Can you work these out from the model? Positions are in its coordinate system, mm. A direction names the side the tool comes from. Round coordinates to 2 decimals unless told otherwise and drop trailing zeros. Write item = value, one per line. Start each with the question number.
1) For faces 1 (the face through (247.476, 9.578, 6.084)), 2 (the face through (77.476, 9.578, 6.084)), which set-ups out of +Z, -Z, +X, -X, +Y, -Y let a thin tool reach every point of the face, with its end or its side?
2) If I drill on line 1 (Y direction, x = 140, z = 6), over which ranges is the centre line in solid material (lowest first)?
3) Thinking about a two-plate mould opening in Z: for faces 3 (the face through (222.558, 9.672, 6.084)), 4 (the face through (123, 5, 12)), which applies, +Z half, -Z half, draft (parallel to the pull), parting line (faces both ways), or undercut?
4) I'm going to push flat-ended pins straight in: pin 1 (0.8 mm diameter, centred on x = 240, z = 3.5, fed in from +Y); pin 2 (1.5 mm diameter, centred on x = 29.5, y = 11, fed in from +Z). Where does each tip first touch, or does it pass through?
5) Imagine slicing it at A-A, the plane y = 8.25. State how many separate pieces and enclosed holes the cut face has, then the cut area to 3 significant figures.
from build123d import *

# Parameters (mm, degrees)
ESBO_O1_W                = 250
ESBO_O1_H                = 13
RESSALTO_EXTRUS_O1_DEPTH = 12
CORTE_EXTRUS_O1_DEPTH    = 251.625218204
PADR_O_LINEAR1_COUNT     = 28
PADR_O_LINEAR1_PITCH     = 10


with BuildPart() as part:
    # Esboço1 → Ressalto-extrusão1 (new body)
    with BuildSketch(Plane.XY):
        with Locations((125, 6.5)):
            Rectangle(ESBO_O1_W, ESBO_O1_H)
    extrude(amount=RESSALTO_EXTRUS_O1_DEPTH)

    # Esboço2 → Corte-extrusão1 (cut, through all)
    with BuildSketch(Plane.XY.offset(12)):
        Polygon((1.312306109, 6.25), (-1.312306109, 6.25), (-3.778350034, 13.0254), (3.778350034, 13.0254), align=None)
    corte_extrus_o1 = extrude(amount=-CORTE_EXTRUS_O1_DEPTH, mode=Mode.SUBTRACT)

    # Padrão linear1: Corte-extrusão1 ×28
    with Locations(*[(i * PADR_O_LINEAR1_PITCH, 0, 0) for i in range(1, PADR_O_LINEAR1_COUNT)]):
        add(corte_extrus_o1, mode=Mode.SUBTRACT)


solid = part.part
Reported:
q1.face_1 = +Z, -Z, +X, +Y
q1.face_2 = +Z, -Z, +Y
q2.line_1 = 0 to 6.25
q3.face_3 = draft
q3.face_4 = +Z half
q4.pin_1 = 6.25
q4.pin_2 = through
q5.separate_pieces = 25
q5.enclosed_holes = 0
q5.area = 1,780 mm²
